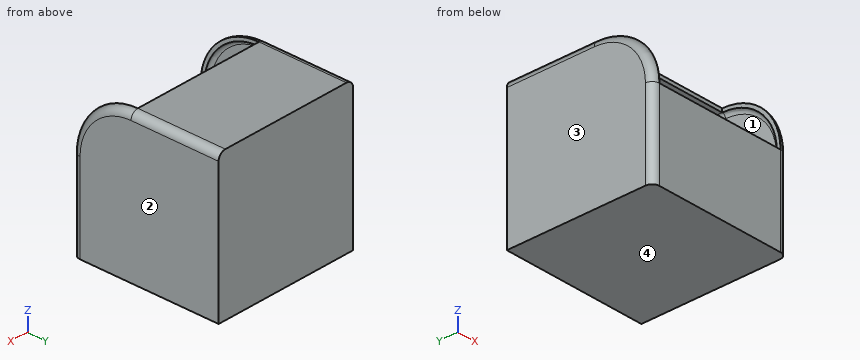
from build123d import *

# Parameters (mm, degrees)
F0_W     = 100
F0_H     = 100
F1_DEPTH = 100
F2_R     = 40
F3_R     = 5
F4_T     = 2.5


# Not quite as in the source:
# - a shell that OpenCascade refuses in one call is made with other operations: the cavity is built on its own and cut out


with BuildPart() as f1:
    # F0 (on Top) → F1 (new body)
    with BuildSketch(Plane.XY):
        Rectangle(F0_W, F0_H)
    extrude(amount=F1_DEPTH)

    # F2
    f2_edges = [f1.edges().sort_by_distance(p)[0] for p in [
        (0, -50, 100),
    ]]
    fillet(f2_edges, radius=F2_R)

    # F3
    f3_edges = [f1.edges().sort_by_distance(p)[0] for p in [
        (50, 20, 100),
        (-50, 20, 100),
    ]]
    fillet(f3_edges, radius=F3_R)

    # F4: shell of thickness 2.5, made by hand


with BuildPart() as f4_core1:
    # F4_t2: copy of F1
    add(f1.part)

    # the walls: a layer under each face that stays
    f4_faces = [f4_core1.faces().sort_by_distance(p)[0] for p in [
        (0, -50, 30),
        (-48.5355339059, -48.5355339059, 30),
        (48.5355339059, -48.5355339059, 30),
        (0, 0, 0),
        (-48.5355339059, -37.2487373415, 87.2487373415),
        (48.5355339059, -37.2487373415, 87.2487373415),
        (0, 20, 100),
        (-50, 2.5, 47.5),
        (50, 2.5, 47.5),
        (0, 50, 50),
        (-48.5355339059, 20, 98.5355339059),
        (48.5355339059, 20, 98.5355339059),
    ]]
    thicken(f4_faces, amount=-F4_T, mode=Mode.SUBTRACT)


with BuildPart() as f1_1:
    add(f1.part)

    # what is left inside the walls is the cavity
    f4_cavity = [f4_core1.part.solids().sort_by_distance(p)[0] for p in [
        (0, -15.833333, 2.525),
    ]]
    add(f4_cavity, mode=Mode.SUBTRACT)


solid = f1_1.part
Geometry: final body of the model. Coordinates: model frame, mm. Face numbers are marked on the shaded views. Give positions to 0.01 mm unless a question says otherwise; leave off trailing zeros. Order: outer loops, then holes, each group sorted by start corner. A loop starts at its lowest first (then second) coordinate and runs counter-clockwise, first axis right, second up. Notation, with made-up numbers: (-10, 54.5) -> (22, 54.5) arc R10 ccw to (22, 61.5) -> close; hole circle Ø1 at (-7.75, -34.75). An arc over 180 degrees is marked (long way). Write each question's results on one line, items separated by ' | '.
1) First-contact query: pin 1 Ø1.2 at (x, z) = (-19, 99) entering from -Y; pin 2 Ø1.3 at (x, y) = (-7, -49.5) entering from +Z; pin 3 Ø3 at (x, y) = (-17.5, -18) entering from +Z. Flat tips, straight axial feed; report the tip coordinate or a pass-through.
Geometry says:
pin 1: stops at y = -10 | pin 2: stops at z = 60 | pin 3: stops at z = 2.5
2) Cut plane A-A (z = 38). Output: boundary loops of the cut face in (x, y), and give its area (3 significant figures).
Geometry says:
outline: (-50, -45) arc R5 ccw to (-45, -50) -> (45, -50) arc R5 ccw to (50, -45) -> (50, 50) -> (-50, 50) -> close; hole (-47.5, -45) arc R2.5 ccw to (-45, -47.5) -> (45, -47.5) arc R2.5 ccw to (47.5, -45) -> (47.5, 47.5) -> (-47.5, 47.5) -> close | area: 967 mm²
3) Cut plane B-B (y = 41). Output: boundary loops of the cut face in (x, z), and give its area (3 significant figures).
Geometry says:
outline: (-50, 0) -> (50, 0) -> (50, 95) arc R5 ccw to (45, 100) -> (-45, 100) arc R5 ccw to (-50, 95) -> close; hole (-47.5, 2.5) -> (47.5, 2.5) -> (47.5, 95) arc R2.5 ccw to (45, 97.5) -> (-45, 97.5) arc R2.5 ccw to (-47.5, 95) -> close | area: 967 mm²
4) Cut plane C-C (x = 31.5). Output: boundary loops of the cut face in (y, z), and give its area (3 significant figures).
Geometry says:
outline: (-50, 0) -> (50, 0) -> (50, 100) -> (-10, 100) -> (-10, 97.5) -> (47.5, 97.5) -> (47.5, 2.5) -> (-47.5, 2.5) -> (-47.5, 60) -> (-50, 60) -> close | area: 781 mm²
5) Line query: line 1 along Y through (x, z) = (-12, 4.5); line 2 along Z through (x, y) = (-38.5, 39). Output: solid intervals per line, ascending.
Geometry says:
line 1: y = -50 to -47.5, 47.5 to 50 | line 2: z = 0 to 2.5, 97.5 to 100
6) Draft query along X for the marked faces 1, 2, 3 and 4. Return one class per face: released by +X, released by -X, zero draft, split by the parting line, or undercut.
Geometry says:
face 1: undercut | face 2: released by +X | face 3: released by -X | face 4: zero draft
